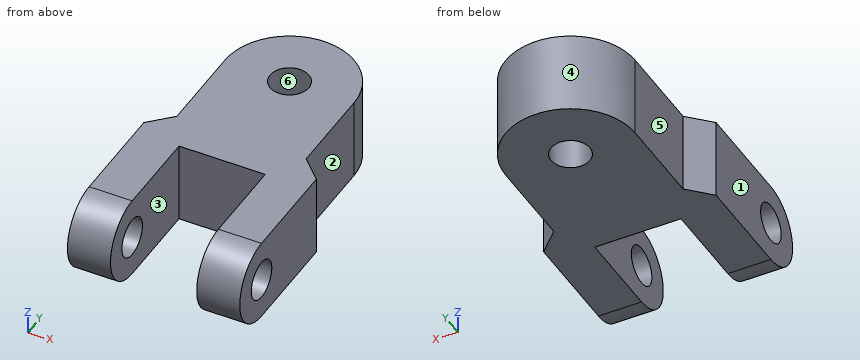
```python
from build123d import *

# Parameters (mm, degrees)
SKETCH1_R                = 2.25
BOSS_EXTRUDE1_DEPTH      = 9.5
BOSS_EXTRUDE2_DEPTH      = 10
BOSS_EXTRUDE2_DEPTH_BACK = 10
SKETCH2_R                = 2.25
SKETCH4_W                = 10
SKETCH4_H                = 15
CUT_EXTRUDE1_DEPTH       = 25.986246217
CHAMFER1_SIZE            = 3


with BuildPart() as part:
    # Sketch1 → Boss-Extrude1 (new body)
    with BuildSketch(Plane.XY):
        with BuildLine():
            Line((0, 0), (15, 0))
            Line((15, 0), (15, 10))
            ThreePointArc((15, 10), (7.5, 17.5), (0, 10))
            Line((0, 10), (0, 0))
        make_face()
        with Locations((7.5, 10)):
            Circle(SKETCH1_R, mode=Mode.SUBTRACT)
    extrude(amount=BOSS_EXTRUDE1_DEPTH)

    # Sketch2 → Boss-Extrude2 (add, two sides: drawn at the far end of the back side and taken through both)
    with BuildSketch(Plane(origin=(7.5, 0, 0), x_dir=(0, 0, -1), z_dir=(1, 0, 0)).offset(-BOSS_EXTRUDE2_DEPTH_BACK)):
        with BuildLine():
            Line((-9.5, 0), (-9.5, -15))
            ThreePointArc((-9.5, -15), (-4.75, -19.75), (0, -15))
            Line((0, -15), (0, 0))
            Line((0, 0), (-9.5, 0))
        make_face()
        with Locations((-4.75, -15)):
            Circle(SKETCH2_R, mode=Mode.SUBTRACT)
    extrude(amount=BOSS_EXTRUDE2_DEPTH + BOSS_EXTRUDE2_DEPTH_BACK)

    # Sketch4 → Cut-Extrude1 (cut, through all)
    with BuildSketch(Plane(origin=(5.5, 0, 9.5), x_dir=(-1, 0, 0), z_dir=(0, 0, -1))):
        with Locations((-2, -12.25)):
            Rectangle(SKETCH4_W, SKETCH4_H)
    extrude(amount=CUT_EXTRUDE1_DEPTH, mode=Mode.SUBTRACT)

    # Chamfer1
    # the kernel refuses this chamfer: 3 mm, written as the material it takes off along each edge
    with BuildSketch(Plane(origin=(-2.5, 0, -7.715048964), x_dir=(0.9996219169112968, 0.027495876610586372, 0), z_dir=(0, 0, 1))) as chamfer1_piece_1_section:
        Polygon((CHAMFER1_SIZE * 0.999621916911, -CHAMFER1_SIZE * 0.0274958766106), (-CHAMFER1_SIZE * 0.0274958766106, -CHAMFER1_SIZE * 0.999621916911), (0, 0), align=None)
    chamfer1_piece_1 = extrude(amount=24.930097928, mode=Mode.PRIVATE)
    chamfer1_piece_1 = split(chamfer1_piece_1, bisect_by=Plane(origin=(0, -1.026079574, 4.75), z_dir=(-1, 0, 0)), keep=Keep.TOP, mode=Mode.PRIVATE)
    add(chamfer1_piece_1, mode=Mode.SUBTRACT)
    with BuildSketch(Plane(origin=(17.5, 0, -7.715048964), x_dir=(0.027495876610586778, -0.9996219169112968, 0), z_dir=(0, 0, 1))) as chamfer1_piece_2_section:
        Polygon((CHAMFER1_SIZE * 0.999621916911, -CHAMFER1_SIZE * 0.0274958766106), (-CHAMFER1_SIZE * 0.0274958766106, -CHAMFER1_SIZE * 0.999621916911), (0, 0), align=None)
    chamfer1_piece_2 = extrude(amount=24.930097928, mode=Mode.PRIVATE)
    chamfer1_piece_2 = split(chamfer1_piece_2, bisect_by=Plane(origin=(15, -1.026079574, 4.75), z_dir=(1, 0, 0)), keep=Keep.TOP, mode=Mode.PRIVATE)
    add(chamfer1_piece_2, mode=Mode.SUBTRACT)


solid = part.part
```
The model under review builds one solid part; all positions refer to its coordinate system, in mm. Face numbers are marked on the shaded views. A direction names the side the tool comes from. Coordinates: 2 decimals unless noted, no trailing zeros. Write each loop counter-clockwise with the first axis right and the second up, starting at its lowest first coordinate (ties: lowest second). Pieces come first, ordered by that corner, then holes. Notation, with made-up numbers: (58.5, 70) -> (105.5, 70) arc R19 ccw to (105.5, 79) -> close; hole circle Ø2 at (-34.5, -16.5). An arc over 180 degrees is marked (long way). One line per item, written item: value. Start each with the question number.
Q1. For the marked faces 1, 2 and 3, list the 3-axis set-ups (+Z, -Z, +X, -X, +Y, -Y) from which the entire face can be reached by the end or side of a thin tool; tool diameter is ignored.
Q2. The part is to be moulded in two halves that separate along X. For the marked faces 4, 5 and 6, say which applies: +X half, -X half, draft (parallel to the pull), parting line (faces both ways), or undercut.
Q3. Add section D-D, the plane z = 8. Give the boundary of the cut face in (x, y).
Q4. Add section C-C, the plane x = 9.25. Give the boundary of the cut face in (y, z), then the cut area to 3 significant figures.
Q5. Clearance check with flat-ended pins moving along their axes: P1, Ø4, axis at x = 1, z = 1.5, coming from the +Y side; P2, Ø3, axis at x = 3.5, z = 4.5, coming from the +Y side; P3, Ø3.5, axis at y = -15, z = 4.75, coming from the -X side; P4, Ø4, axis at y = 7, z = 4, coming from the +X side. State where each tip first meets the part, or that it passes through.
Q6. Add section A-A, the plane z = 4.75. Give the boundary of the cut face in (x, y).
Q7. Add section B-B, the plane y = -8. Give the boundary of the cut face in (x, z), then the cut area to 3 significant figures.
Q8. To check wall thickness, follow probe 1 along X at (y, z) = (-10.5, 6.5); probe 2 along Y at (x, z) = (7.5, 3.5); probe 3 along Z at (x, y) = (13.6, -15). State the ranges of each line that lie inside material, in increasing order.
Response:
1. face 1: +Z, -Z, -X, +Y, -Y
1. face 2: +Z, -Z, +X, +Y
1. face 3: +Z, -Z, -Y
2. face 4: parting line
2. face 5: -X half
2. face 6: undercut
3. outline: (-2.5, -18.46) -> (2.5, -18.46) -> (2.5, -4.75) -> (12.5, -4.75) -> (12.5, -18.46) -> (17.5, -18.46) -> (17.5, -3) -> (15, -0.5) -> (15, 10) arc R7.5 ccw to (0, 10) -> (0, -0.5) -> (-2.5, -3) -> close; hole circle Ø4.5 at (7.5, 10)
4. outline: (-4.75, 0) -> (8.59, 0) -> (8.59, 9.5) -> (-4.75, 9.5) -> close; (11.41, 0) -> (17.29, 0) -> (17.29, 9.5) -> (11.41, 9.5) -> close
4. area: 183 mm²
5. P1: y = 16
5. P2: y = 17.07
5. P3: through
5. P4: x = 15
6. outline: (-2.5, -19.75) -> (2.5, -19.75) -> (2.5, -17.25) -> (-2.5, -17.25) -> close; (-2.5, -12.75) -> (2.5, -12.75) -> (2.5, -4.75) -> (12.5, -4.75) -> (12.5, -12.75) -> (17.5, -12.75) -> (17.5, -3) -> (15, -0.5) -> (15, 10) arc R7.5 ccw to (0, 10) -> (0, -0.5) -> (-2.5, -3) -> close; (12.5, -19.75) -> (17.5, -19.75) -> (17.5, -17.25) -> (12.5, -17.25) -> close; hole circle Ø4.5 at (7.5, 10)
7. outline: (-2.5, 0) -> (2.5, 0) -> (2.5, 9.5) -> (-2.5, 9.5) -> close; (12.5, 0) -> (17.5, 0) -> (17.5, 9.5) -> (12.5, 9.5) -> close
7. area: 95.0 mm²
8. probe 1: -2.5 to 2.5, 12.5 to 17.5
8. probe 2: -4.75 to 7.75, 12.25 to 17.5
8. probe 3: 0 to 2.5, 7 to 9.5
